Read the model definition and answer for the solid it produces. Units are mm, in the model's axes. A direction names the side the tool comes from. Round coordinates to 2 decimals unless told otherwise and drop trailing zeros. Loops run counter-clockwise (first coordinate to the right, second up) from the corner with the lowest first, then second, coordinate; pieces in that order, holes last. Notation, with made-up numbers: (60.25, -20) - (110.25, -20) arc R19 cw to (110.25, 6) - close; hole circle Ø5 at (2, 60.5). An arc over 180 degrees is marked (long way). Use CSV: the item, a comma, the result in double quotes. Start each with the question number.
1. Find section B-B (x = 0). Give the vertices of the cut face in (y, z) (3 decimals), and give its area (3 significant figures).
2. Find section A-A (z = 0). Give the vertices of the cut face in (x, y) (3 decimals).
3. Find section D-D (y = 30). Give the vertices of the cut face in (x, z) (3 decimals).
4. A tool of negligible diameter and unlimited length cuts with its end or side. For faces 4 (the flat face through (3, 55, -2)), 5 (the cylindrical face through (5.158, 29.65, 3.955)), from which of +Z, -Z, +X, -X, +Y, -Y can it reach the whole face along a straight path? Write none if from no direction.
5. Determine the mould class of faces 1 (the flat face through (-5, 5, -5)), 2 (the flat face through (0, 0, 5)), 3 (the conical face through (-10.742, 8.712, 20.653)) for opening direction X: +X half, -X half, draft (parallel to the pull), parting line (faces both ways), or undercut.
6. Consider line 1 along Z through (x, y) = (0, 32) (3 decimals); line 2 along Z through (x, y) = (0, 6) (3 decimals); line 3 along Z through (x, y) = (0, 7) (1 decimal). Determine where each line is inside the solid, lowest interval first.
7. Given pin 1 Ø6 at (y, z) = (12.5, 16) entering from -X; pin 2 Ø10 at (x, y) = (6.5, 30) entering from -Z; pin 3 Ø10 at (y, z) = (5.5, -18.5) entering from -X, each flat-ended and moving along its own axis, determine where each tip first touches the part or whether it passes through.
8. Find section C-C (y = 6). Give the vertices of the cut face in (x, z) (3 decimals), and give its area (3 significant figures).
from build123d import *

# Parameters (mm, degrees)
F2_R = 1


with BuildPart() as f1:
    # F0 (on Top) → F1 (revolve)
    with BuildSketch(Plane.XY):
        Polygon((-25.175, 0), (-3.175, 0), (-3.175, 55), (-6.5, 55), (-6.5, 5), (-20, 5), (-20, 10), (-23, 10), align=None)
    revolve(axis=Axis((0, 30.933686, 0), (0, -1, 0)))

    # F2
    f2_edges = [f1.edges().sort_by_distance(p)[0] for p in [
        (25.175, 0, 0),
        (23, 10, 0),
        (20, 10, 0),
    ]]
    fillet(f2_edges, radius=F2_R)


solid = f1.part
Filled sheet:
1,outline,"(0, -23.934) arc R1 ccw to (1.213, -24.911) - (9.213, -23.171) arc R1 ccw to (10, -22.194) - (10, -21) arc R1 ccw to (9, -20) - (5, -20) - (5, -6.5) - (55, -6.5) - (55, -3.175) - (0, -3.175) - close; (0, 3.175) - (55, 3.175) - (55, 6.5) - (5, 6.5) - (5, 20) - (9, 20) arc R1 ccw to (10, 21) - (10, 22.194) arc R1 ccw to (9.213, 23.171) - (1.213, 24.911) arc R1 ccw to (0, 23.934) - close"
1,area,"581 mm²"
2,outline,"(-24.911, 1.213) arc R1 ccw to (-23.934, 0) - (-3.175, 0) - (-3.175, 55) - (-6.5, 55) - (-6.5, 5) - (-20, 5) - (-20, 9) arc R1 ccw to (-21, 10) - (-22.194, 10) arc R1 ccw to (-23.171, 9.213) - close; (3.175, 0) - (23.934, 0) arc R1 ccw to (24.911, 1.213) - (23.171, 9.213) arc R1 ccw to (22.194, 10) - (21, 10) arc R1 ccw to (20, 9) - (20, 5) - (6.5, 5) - (6.5, 55) - (3.175, 55) - close"
3,outline,"circle Ø13 at (0, 0); hole circle Ø6.35 at (0, 0)"
4,face 4,"+Z, -Z, +X, -X, +Y"
4,face 5,"+Y"
5,face 1,"undercut"
5,face 2,"draft"
5,face 3,"parting line"
6,line 1,"z = -6.5 to -3.175, 3.175 to 6.5"
6,line 2,"z = -23.87 to -20, -6.5 to -3.175, 3.175 to 6.5, 20 to 23.87"
6,line 3,"z = -23.7 to -20, -6.5 to -3.2, 3.2 to 6.5, 20 to 23.7"
7,pin 1,"stops at x = -17.43"
7,pin 2,"stops at z = -6.32"
7,pin 3,"stops at x = -20.06"
8,outline,"circle Ø47.74 at (0, 0); circle Ø13 at (0, 0); hole circle Ø40 at (0, 0); hole circle Ø6.35 at (0, 0)"
8,area,"634 mm²"
